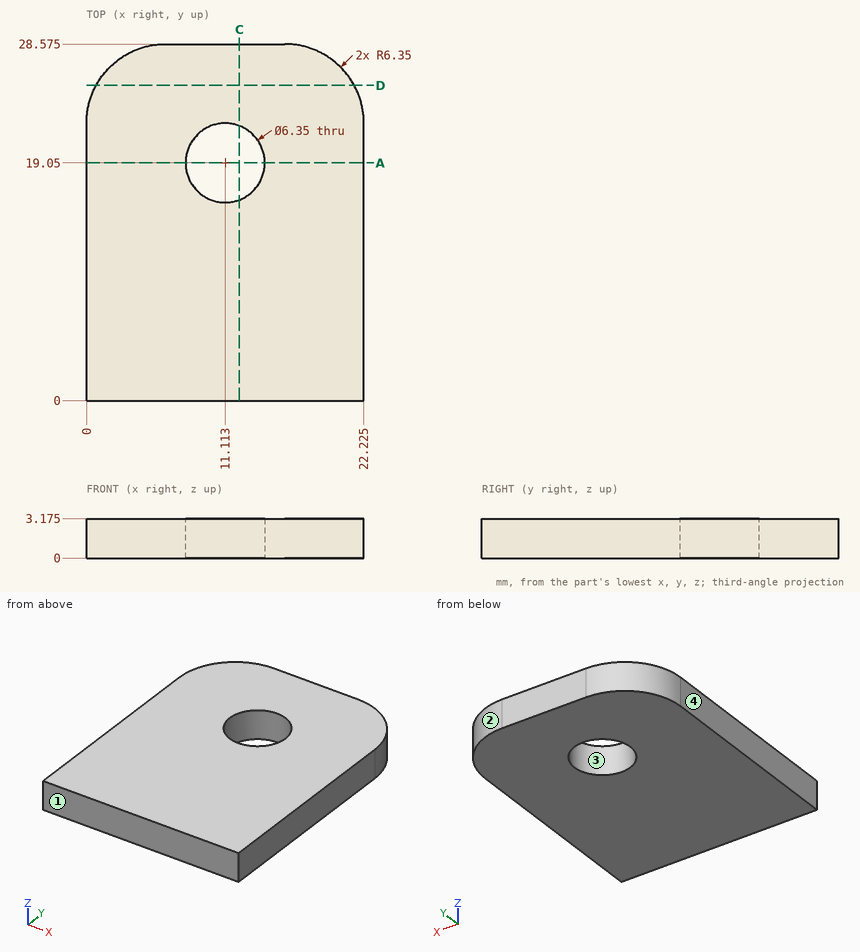
Could you check a few things on this drawing? It's one solid part, dimensions in mm from its lowest x, y, z. Round coordinates to 2 decimals unless told otherwise and drop trailing zeros. Order: outer loops, then holes, each group sorted by start corner. A loop starts at its lowest first (then second) coordinate and runs counter-clockwise, first axis right, second up.
(1) I'm going to push a flat-ended pin straight in: pin 1 (5 mm diameter, centred on x = 11.11, y = 19.05, fed in from -Z). Where does the tip first touch, or does it pass through?
Response values:
pin 1: passes through
(2) Imagine slicing it at D-D (y = 25.25). Write out the boundary of the cut face in (x, z) (1 decimal).
Response values:
outline: (0.8, 0) - (21.5, 0) - (21.5, 3.2) - (0.8, 3.2) - close
(3) Please list where these lines run through material, in increasing order: line 1 along Y through (x, z) = (11.25, 2.65) (1 decimal); line 2 along X through (y, z) = (16.75, 0.15) (1 decimal); line 3 along X through (y, z) = (20.5, 2.3) (1 decimal).
Response values:
line 1: y = 0 to 15.9, 22.2 to 28.6
line 2: x = 0 to 8.9, 13.3 to 22.2
line 3: x = 0 to 8.3, 13.9 to 22.2
(4) Imagine slicing it at C-C (x = 12.25). Write out the boundary of the cut face in (y, z) (1 decimal).
Response values:
outline: (0, 0) - (16.1, 0) - (16.1, 3.2) - (0, 3.2) - close; (22, 0) - (28.6, 0) - (28.6, 3.2) - (22, 3.2) - close
(5) If we mould it in two halves opening along X, with no side actions, what happens to the marked faces 1, 2, 3 and 4? For each: released by +X, released by -X, zero draft, split by the parting line, or undercut.
Response values:
face 1: zero draft
face 2: released by +X
face 3: undercut
face 4: released by -X
(6) Imagine slicing it at A-A (y = 19.05). Write out the boundary of the cut face in (x, z) (1 decimal).
Response values:
outline: (0, 0) - (7.9, 0) - (7.9, 3.2) - (0, 3.2) - close; (14.3, 0) - (22.2, 0) - (22.2, 3.2) - (14.3, 3.2) - close
